Work out the finished part from the listing and answer in its coordinate system (mm). Coordinates: 2 decimals unless noted, no trailing zeros. Order: outer loops, then holes, each group sorted by start corner. A loop starts at its lowest first (then second) coordinate and runs counter-clockwise, first axis right, second up. Notation, with made-up numbers: M 27,-40 L 48,-40 A23 cw 48,-4 Z; hole C 2.5,76.25 d10. An arc over 180 degrees is marked long. Use a Markdown table: item, result.
from build123d import *

# Parameters (mm, degrees)
F0_W         = 15.2291797996
F0_H         = 88.5
F0_W_2       = 14.7708202004
F1_DEPTH     = 1.5
F2_T1_DEPTH  = 88.5
F2_T3_DEPTH  = 156
F2_T9_DEPTH  = 93.3412291828
F2_T13_DEPTH = 160.8412291828
F2_T20_DEPTH = 93.3412291828
F2_T24_DEPTH = 160.8412291828
F2_T31_DEPTH = 160.8412291828
F2_T35_DEPTH = 93.3412291828
F2_T42_DEPTH = 93.3412291828
F2_T46_DEPTH = 160.8412291828
F3_T1_DEPTH  = 203.8535710714
F3_T3_DEPTH  = 136.3535710714


# Not quite as in the source:
# - a fillet or chamfer that OpenCascade refuses, or shapes differently, is made with other operations: its cross-section is extruded or revolved along the edge and cut away or added


with BuildPart() as f1:
    # F0 (on Front) → F1 (new body)
    with BuildSketch(Plane.XZ):
        with Locations((-70.9603581131, 10.6903343201)):
            Rectangle(F0_W, F0_H)
        with Locations((100.0396418869, 10.6903343201)):
            Rectangle(F0_W_2, F0_H)
        Polygon((-78.5749480128, 54.9403343201), (-63.3457682133, 54.9403343201), (92.4250519872, 54.9403343201), (92.6542317867, 54.9403343201), (107.4250519872, 54.9403343201), (107.4250519872, 69.9403343201), (107.4249148369, 69.9403343201), (92.6542317867, 69.9403343201), (-63.3457682133, 69.9403343201), (-78.5749480128, 69.9403343201), (-78.5749480128, 64.060893178), align=None)
        Polygon((92.6542317867, -33.5596656799), (-63.3457682133, -33.5596656799), (-78.5749480128, -33.5596656799), (-78.5749480128, -40.4141508043), (-78.5749480128, -48.5596656799), (-63.5749480128, -48.5596656799), (-63.3457682133, -48.5596656799), (92.6542317867, -48.5596656799), (107.4250519872, -48.5596656799), (107.4250519872, -33.5596656799), align=None)
    extrude(amount=F1_DEPTH)

    # F2: fillet of radius 2 on 4 edges, made by hand

    # F2_s2 → F2_t1 (cut)
    with BuildSketch(Plane.XY.offset(-33.5596656799)):
        with BuildLine():
            ThreePointArc((-63.3457682133, 0), (-64.057515015, -1.0811388301), (-65.2822598864, -1.5))
            Line((-65.2822598864, -1.5), (-63.3457682133, -1.5))
            Line((-63.3457682133, -1.5), (-63.3457682133, 0))
        make_face()
        with BuildLine():
            ThreePointArc((92.6542317867, 0), (93.3659785884, -1.0811388301), (94.5907234598, -1.5))
            Line((94.5907234598, -1.5), (92.6542317867, -1.5))
            Line((92.6542317867, -1.5), (92.6542317867, 0))
        make_face()
    extrude(amount=F2_T1_DEPTH, mode=Mode.SUBTRACT)

    # F2_s4 → F2_t3 (cut)
    with BuildSketch(Plane.YZ.offset(-63.3457682133)):
        with BuildLine():
            ThreePointArc((0, 54.9403343201), (-1.0811388301, 55.6520811218), (-1.5, 56.8768259932))
            Line((-1.5, 56.8768259932), (-1.5, 54.9403343201))
            Line((-1.5, 54.9403343201), (0, 54.9403343201))
        make_face()
        with BuildLine():
            ThreePointArc((0, -33.5596656799), (-1.0811388301, -34.2714124816), (-1.5, -35.496157353))
            Line((-1.5, -35.496157353), (-1.5, -33.5596656799))
            Line((-1.5, -33.5596656799), (0, -33.5596656799))
        make_face()
    extrude(amount=F2_T3_DEPTH, mode=Mode.SUBTRACT)


with BuildPart() as f2_tool7:
    # F2_s8 → F2_t9 (new body)
    with BuildSketch(Plane.XY.offset(-38.4008948627)):
        with BuildLine():
            ThreePointArc((-63.3457682133, 0), (-64.057515015, -1.0811388301), (-65.2822598864, -1.5))
            Line((-65.2822598864, -1.5), (-63.3457682133, -1.5))
            Line((-63.3457682133, -1.5), (-63.3457682133, 0))
        make_face()
    extrude(amount=F2_T9_DEPTH)

    split(bisect_by=Plane.XY.offset(-33.5596656799), keep=Keep.BOTTOM)


with BuildPart() as f2_tool11:
    # F2_s12 → F2_t13 (new body)
    with BuildSketch(Plane.YZ.offset(92.6542317867)):
        with BuildLine():
            ThreePointArc((0, -33.5596656799), (-1.0811388301, -34.2714124816), (-1.5, -35.496157353))
            Line((-1.5, -35.496157353), (-1.5, -33.5596656799))
            Line((-1.5, -33.5596656799), (0, -33.5596656799))
        make_face()
    extrude(amount=-F2_T13_DEPTH)

    split(bisect_by=Plane.YZ.offset(-63.3457682133), keep=Keep.BOTTOM)


with BuildPart() as f2_tool7_1:
    add(f2_tool7.part)

    # F2_t15: intersect F2_tool11
    add(f2_tool11.part, mode=Mode.INTERSECT)


with BuildPart() as f1_1:
    add(f1.part)

    # F2_t5: cut F2_tool7
    add(f2_tool7_1.part, mode=Mode.SUBTRACT)


with BuildPart() as f2_tool18:
    # F2_s19 → F2_t20 (new body)
    with BuildSketch(Plane.XY.offset(-33.5596656799)):
        with BuildLine():
            ThreePointArc((-63.3457682133, 0), (-64.057515015, -1.0811388301), (-65.2822598864, -1.5))
            Line((-65.2822598864, -1.5), (-63.3457682133, -1.5))
            Line((-63.3457682133, -1.5), (-63.3457682133, 0))
        make_face()
    extrude(amount=F2_T20_DEPTH)

    split(bisect_by=Plane.XY.offset(54.9403343201), keep=Keep.TOP)


with BuildPart() as f2_tool22:
    # F2_s23 → F2_t24 (new body)
    with BuildSketch(Plane.YZ.offset(-68.186997396)):
        with BuildLine():
            ThreePointArc((0, 54.9403343201), (-1.0811388301, 55.6520811218), (-1.5, 56.8768259932))
            Line((-1.5, 56.8768259932), (-1.5, 54.9403343201))
            Line((-1.5, 54.9403343201), (0, 54.9403343201))
        make_face()
    extrude(amount=F2_T24_DEPTH)

    split(bisect_by=Plane.YZ.offset(-63.3457682133), keep=Keep.BOTTOM)


with BuildPart() as f2_tool18_1:
    add(f2_tool18.part)

    # F2_t26: intersect F2_tool22
    add(f2_tool22.part, mode=Mode.INTERSECT)


with BuildPart() as f1_2:
    add(f1_1.part)

    # F2_t16: cut F2_tool18
    add(f2_tool18_1.part, mode=Mode.SUBTRACT)


with BuildPart() as f2_tool29:
    # F2_s30 → F2_t31 (new body)
    with BuildSketch(Plane.YZ.offset(-63.3457682133)):
        with BuildLine():
            ThreePointArc((0, 54.9403343201), (-1.0811388301, 55.6520811218), (-1.5, 56.8768259932))
            Line((-1.5, 56.8768259932), (-1.5, 54.9403343201))
            Line((-1.5, 54.9403343201), (0, 54.9403343201))
        make_face()
    extrude(amount=F2_T31_DEPTH)

    split(bisect_by=Plane.YZ.offset(92.6542317867), keep=Keep.TOP)


with BuildPart() as f2_tool33:
    # F2_s34 → F2_t35 (new body)
    with BuildSketch(Plane.XY.offset(59.7815635028)):
        with BuildLine():
            ThreePointArc((92.6542317867, 0), (93.3659785884, -1.0811388301), (94.5907234598, -1.5))
            Line((94.5907234598, -1.5), (92.6542317867, -1.5))
            Line((92.6542317867, -1.5), (92.6542317867, 0))
        make_face()
    extrude(amount=-F2_T35_DEPTH)

    split(bisect_by=Plane.XY.offset(54.9403343201), keep=Keep.TOP)


with BuildPart() as f2_tool29_1:
    add(f2_tool29.part)

    # F2_t37: intersect F2_tool33
    add(f2_tool33.part, mode=Mode.INTERSECT)


with BuildPart() as f1_3:
    add(f1_2.part)

    # F2_t27: cut F2_tool29
    add(f2_tool29_1.part, mode=Mode.SUBTRACT)


with BuildPart() as f2_tool40:
    # F2_s41 → F2_t42 (new body)
    with BuildSketch(Plane.XY.offset(54.9403343201)):
        with BuildLine():
            ThreePointArc((92.6542317867, 0), (93.3659785884, -1.0811388301), (94.5907234598, -1.5))
            Line((94.5907234598, -1.5), (92.6542317867, -1.5))
            Line((92.6542317867, -1.5), (92.6542317867, 0))
        make_face()
    extrude(amount=-F2_T42_DEPTH)

    split(bisect_by=Plane.XY.offset(-33.5596656799), keep=Keep.BOTTOM)


with BuildPart() as f2_tool44:
    # F2_s45 → F2_t46 (new body)
    with BuildSketch(Plane.YZ.offset(97.4954609695)):
        with BuildLine():
            ThreePointArc((0, -33.5596656799), (-1.0811388301, -34.2714124816), (-1.5, -35.496157353))
            Line((-1.5, -35.496157353), (-1.5, -33.5596656799))
            Line((-1.5, -33.5596656799), (0, -33.5596656799))
        make_face()
    extrude(amount=-F2_T46_DEPTH)

    split(bisect_by=Plane.YZ.offset(92.6542317867), keep=Keep.TOP)


with BuildPart() as f2_tool40_1:
    add(f2_tool40.part)

    # F2_t48: intersect F2_tool44
    add(f2_tool44.part, mode=Mode.INTERSECT)


with BuildPart() as f1_4:
    add(f1_3.part)

    # F2_t38: cut F2_tool40
    add(f2_tool40_1.part, mode=Mode.SUBTRACT)

    # F3: fillet of radius 5 on 4 edges, made by hand

    # F3_s2 → F3_t1 (cut)
    with BuildSketch(Plane.YZ.offset(-87.5017335485)):
        with BuildLine():
            ThreePointArc((-1.5, 66.3696201058), (-1.1097722286, 68.3061117789), (0, 69.9403343201))
            Line((0, 69.9403343201), (-1.5, 69.9403343201))
            Line((-1.5, 69.9403343201), (-1.5, 66.3696201058))
        make_face()
        with BuildLine():
            ThreePointArc((-1.5, -44.9889514657), (-1.1097722286, -46.9254431388), (0, -48.5596656799))
            Line((0, -48.5596656799), (-1.5, -48.5596656799))
            Line((-1.5, -48.5596656799), (-1.5, -44.9889514657))
        make_face()
    extrude(amount=F3_T1_DEPTH, mode=Mode.SUBTRACT)

    # F3_s4 → F3_t3 (cut)
    with BuildSketch(Plane.XY.offset(-57.4864512156)):
        with BuildLine():
            ThreePointArc((103.8543377729, -1.5), (105.790829446, -1.1097722286), (107.4250519872, 0))
            Line((107.4250519872, 0), (107.4250519872, -1.5))
            Line((107.4250519872, -1.5), (103.8543377729, -1.5))
        make_face()
        with BuildLine():
            ThreePointArc((-75.0042337986, -1.5), (-76.9407254717, -1.1097722286), (-78.5749480128, 0))
            Line((-78.5749480128, 0), (-78.5749480128, -1.5))
            Line((-78.5749480128, -1.5), (-75.0042337986, -1.5))
        make_face()
    extrude(amount=F3_T3_DEPTH, mode=Mode.SUBTRACT)


solid = f1_4.part
(1) A cutting plane is placed at A-A (x = 26). Determine the outline of the cut face in (y, z), then the cut area to 3 significant figures.
Conclusion:
| item | result |
|---|---|
| outline | M -1.5,-44.99 A5 ccw 0,-48.56 L 0,-33.56 A2 ccw -1.5,-35.5 Z; M -1.5,56.88 A2 ccw 0,54.94 L 0,69.94 A5 ccw -1.5,66.37 Z |
| area | 40.2 mm2 |
(2) A cutting plane is placed at B-B (z = -0.5). Determine the outline of the cut face in (x, y).
Conclusion:
| item | result |
|---|---|
| outline | M -78.57,0 A5 ccw -75,-1.5 L -65.28,-1.5 A2 ccw -63.35,0 Z; M 92.65,0 A2 ccw 94.59,-1.5 L 103.85,-1.5 A5 ccw 107.43,0 Z |
(3) Given P1, Ø6, axis at x = 0, z = -29, coming from the -Y side, flat-ended and moving along its own axis, determine where the tip first touches the part or whether it passes through.
Conclusion:
| item | result |
|---|---|
| P1 | through |
(4) A cutting plane is placed at C-C (y = -0.6). Determine the outline of the cut face in (x, z).
Conclusion:
| item | result |
|---|---|
| outline | M -77.87,-47.85 L 106.72,-47.85 L 106.72,69.23 L -77.87,69.23 Z; hole M -63.61,-33.83 L 92.92,-33.83 L 92.92,55.21 L -63.61,55.21 Z |
(5) Straight lines are drawn through the part: L1, parallel to Z at x = 85, y = -0.5; L2, parallel to X at y = -0.85, z = 50.5; L3, parallel to X at y = -0.4, z = 37. For each, find the intervals that lie inside material, in ascending order.
Conclusion:
| item | result |
|---|---|
| L1 | -47.99 to -33.76, 55.14 to 69.37 |
| L2 | -77.47 to -63.81, 93.12 to 106.32 |
| L3 | -78.13 to -63.5, 92.8 to 106.98 |
